Model file for the job. Use its own axes, mm. Face numbers are marked on the shaded views. Coordinates: 2 decimals unless noted, no trailing zeros. Write each loop counter-clockwise with the first axis right and the second up, starting at its lowest first coordinate (ties: lowest second). Pieces come first, ordered by that corner, then holes. Notation, with made-up numbers: (80, 34) -> (106, 34) arc R24 cw to (106, 61) -> close; hole circle Ø8 at (-6, 27.5). An arc over 180 degrees is marked (long way). Write item = value, one per line. Start each with the question number.
from build123d import *

# Parameters (mm, degrees)
SKETCH1_W           = 100
SKETCH1_H           = 120
SKETCH1_R           = 2.5
SKETCH1_R_2         = 7.5
BOSS_EXTRUDE1_DEPTH = 4
CHAMFER1_SIZE       = 10
SKETCH2_R           = 2.5
SKETCH2_R_2         = 4
CUT_EXTRUDE1_DEPTH  = 131.245921241


with BuildPart() as part:
    # Sketch1 → Boss-Extrude1 (new, symmetric)
    with BuildSketch(Plane.XY):
        with Locations((0, 60)):
            Rectangle(SKETCH1_W, SKETCH1_H)
        with Locations((-42, 6.66986634)):
            Circle(SKETCH1_R, mode=Mode.SUBTRACT)
        with Locations((-21, 6.66986634)):
            Circle(SKETCH1_R, mode=Mode.SUBTRACT)
        with Locations((-42, 34.66986634)):
            Circle(SKETCH1_R, mode=Mode.SUBTRACT)
        with Locations((-21, 34.66986634)):
            Circle(SKETCH1_R, mode=Mode.SUBTRACT)
        with Locations((-10.5, 112)):
            Circle(SKETCH1_R, mode=Mode.SUBTRACT)
        with Locations((-10.5, 84)):
            Circle(SKETCH1_R, mode=Mode.SUBTRACT)
        with Locations(Location((10.5, 84, 0), (0, 0, 180))):
            Circle(SKETCH1_R, mode=Mode.SUBTRACT)
        with Locations(Location((10.5, 112, 0), (0, 0, 180))):
            Circle(SKETCH1_R, mode=Mode.SUBTRACT)
        with Locations(Location((21, 34.66986634, 0), (0, 0, 180))):
            Circle(SKETCH1_R, mode=Mode.SUBTRACT)
        with Locations(Location((42, 34.66986634, 0), (0, 0, 180))):
            Circle(SKETCH1_R, mode=Mode.SUBTRACT)
        with Locations(Location((21, 6.66986634, 0), (0, 0, 180))):
            Circle(SKETCH1_R, mode=Mode.SUBTRACT)
        with Locations(Location((42, 6.66986634, 0), (0, 0, 180))):
            Circle(SKETCH1_R, mode=Mode.SUBTRACT)
        with Locations((0, 65)):
            Circle(SKETCH1_R_2, mode=Mode.SUBTRACT)
    extrude(amount=BOSS_EXTRUDE1_DEPTH, both=True)

    # Chamfer1
    chamfer1_edges = [part.edges().sort_by_distance(p)[0] for p in [
        (-50, 120, 0),
        (50, 120, 0),
    ]]
    chamfer(chamfer1_edges, length=CHAMFER1_SIZE)

    # Sketch2 → Cut-Extrude1 (cut, through all)
    with BuildSketch(Plane.XY.offset(4)):
        with Locations((-15.5, 80.98)):
            Circle(SKETCH2_R)
        with Locations((-15.5, 49.98)):
            Circle(SKETCH2_R)
        with Locations((15.5, 80.98)):
            Circle(SKETCH2_R)
        with Locations((15.5, 49.98)):
            Circle(SKETCH2_R)
        with Locations((-34, 51.98)):
            Circle(SKETCH2_R_2)
        with Locations((34, 51.98)):
            Circle(SKETCH2_R_2)
    extrude(amount=-CUT_EXTRUDE1_DEPTH, mode=Mode.SUBTRACT)


solid = part.part
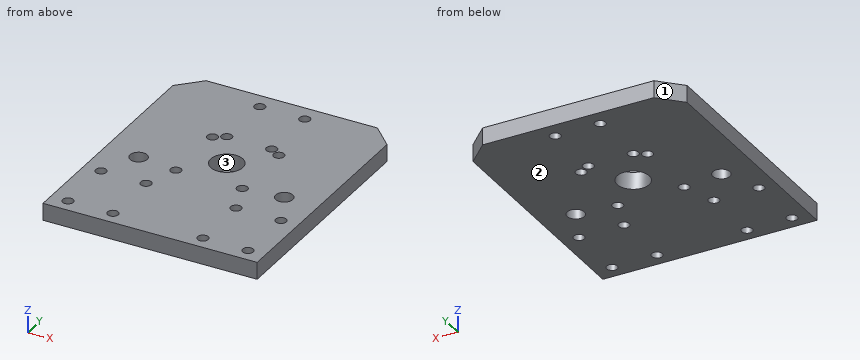
(1) Drill centre lines: line 1 along Y through (x, z) = (15.5, 3.5); line 2 along Y through (x, z) = (21, -1); line 3 along Y through (x, z) = (34, 1). Where is each one in solid material? Low to high.
(2) Saw through at D-D (x = -0.5). Give the cut face in (y, z).
(3) Saw through at C-C (z = 0). State how many separate pieces and enclosed holes the cut face has, then the cut area to 3 significant figures.
(4) Saw through at A-A (y = 65). Give the cut face in (x, z).
(5) Saw through at B-B (x = -15.5). Give the cut face in (y, z).
(6) Mould opens along Y. For the marked faces 1, 2 and 3 say: released by +Y, released by -Y, zero draft, split by the parting line, or undercut.
Returned:
q1.line_1 = 0 to 47.48, 52.48 to 78.48, 83.48 to 120
q1.line_2 = 0 to 4.17, 9.17 to 32.17, 37.17 to 120
q1.line_3 = 0 to 47.98, 55.98 to 120
q2.outline = (0, -4) -> (57.52, -4) -> (57.52, 4) -> (0, 4) -> close; (72.48, -4) -> (120, -4) -> (120, 4) -> (72.48, 4) -> close
q3.separate_pieces = 1
q3.enclosed_holes = 19
q3.area = 11,300 mm2
q4.outline = (-50, -4) -> (-7.5, -4) -> (-7.5, 4) -> (-50, 4) -> close; (7.5, -4) -> (50, -4) -> (50, 4) -> (7.5, 4) -> close
q5.outline = (0, -4) -> (47.48, -4) -> (47.48, 4) -> (0, 4) -> close; (52.48, -4) -> (78.48, -4) -> (78.48, 4) -> (52.48, 4) -> close; (83.48, -4) -> (120, -4) -> (120, 4) -> (83.48, 4) -> close
q6.face_1 = released by +Y
q6.face_2 = zero draft
q6.face_3 = undercut
